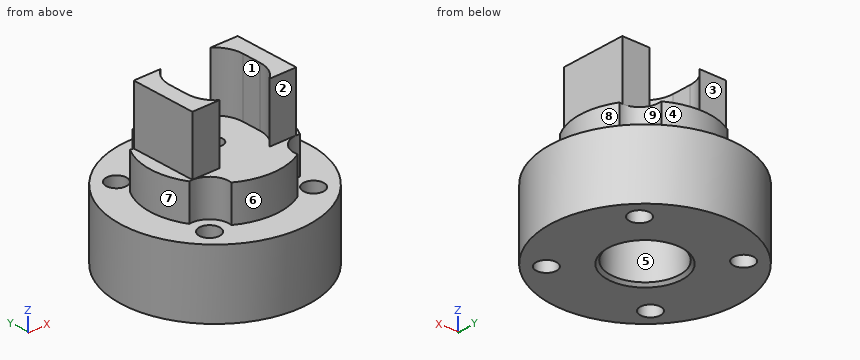
```python
from build123d import *

# Parameters (mm, degrees)
SKIZZE1_R                       = 6.7
AUFSATZ_LINEAR_AUSTRAGEN1_DEPTH = 3.75
SKIZZE1_7_R                     = 9.75
SKIZZE1_7_R_2                   = 3.55
AUFSATZ_LINEAR_AUSTRAGEN2_DEPTH = 7
SKIZZE5_R                       = 1.05
SCHNITT_LINEAR_AUSTRAGEN1_DEPTH = 11.75
SKIZZE5_3_R                     = 2
SKIZZE5_3_R_2                   = 1.05
SCHNITT_LINEAR_AUSTRAGEN2_DEPTH = 3.75
FASE1_SIZE                      = 0.3
AUFSATZ_LINEAR_AUSTRAGEN4_DEPTH = 6
M2_GEWINDEBOHRUNG1_D            = 1.6


with BuildPart() as part:
    # Skizze1 → Aufsatz-Linear austragen1 (new body)
    with BuildSketch(Plane.XY):
        Circle(SKIZZE1_R)
    extrude(amount=AUFSATZ_LINEAR_AUSTRAGEN1_DEPTH)

    # Skizze1<7> → Aufsatz-Linear austragen2 (add)
    with BuildSketch(Plane.XY):
        Circle(SKIZZE1_7_R)
        Circle(SKIZZE1_7_R_2, mode=Mode.SUBTRACT)
    extrude(amount=-AUFSATZ_LINEAR_AUSTRAGEN2_DEPTH)

    # Skizze5 → Schnitt-Linear austragen1 (cut, through all)
    with BuildSketch(Plane.XY.offset(3.75)):
        with Locations((5.409366876, 5.409366876)):
            Circle(SKIZZE5_R)
        with Locations((5.409366876, -5.409366876)):
            Circle(SKIZZE5_R)
        with Locations((-5.409366876, -5.409366876)):
            Circle(SKIZZE5_R)
        with Locations((-5.409366876, 5.409366876)):
            Circle(SKIZZE5_R)
    extrude(amount=-SCHNITT_LINEAR_AUSTRAGEN1_DEPTH, mode=Mode.SUBTRACT)

    # Skizze5<3> → Schnitt-Linear austragen2 (cut)
    with BuildSketch(Plane.XY.offset(3.75)):
        with Locations((-5.409366876, 5.409366876)):
            Circle(SKIZZE5_3_R)
        with Locations((-5.409366876, 5.409366876)):
            Circle(SKIZZE5_3_R_2, mode=Mode.SUBTRACT)
        with Locations((5.409366876, 5.409366876)):
            Circle(SKIZZE5_3_R)
        with Locations((5.409366876, 5.409366876)):
            Circle(SKIZZE5_3_R_2, mode=Mode.SUBTRACT)
        with Locations((5.409366876, -5.409366876)):
            Circle(SKIZZE5_3_R)
        with Locations((5.409366876, -5.409366876)):
            Circle(SKIZZE5_3_R_2, mode=Mode.SUBTRACT)
        with Locations((-5.409366876, -5.409366876)):
            Circle(SKIZZE5_3_R)
        with Locations((-5.409366876, -5.409366876)):
            Circle(SKIZZE5_3_R_2, mode=Mode.SUBTRACT)
    extrude(amount=-SCHNITT_LINEAR_AUSTRAGEN2_DEPTH, mode=Mode.SUBTRACT)

    # Fase1
    fase1_edges = [part.edges().sort_by_distance(p)[0] for p in [
        (-3.55, 0, -7),
    ]]
    chamfer(fase1_edges, length=FASE1_SIZE)

    # Skizze7 → Aufsatz-Linear austragen4 (add)
    with BuildSketch(Plane.XY.offset(3.75)):
        with BuildLine():
            Line((-5.4, 3.4), (-2.6, 3.4))
            ThreePointArc((-2.6, 3.4), (-3.483281573, 2.341640786), (-3.8, 1))
            Line((-3.8, 1), (-3.8, -1))
            ThreePointArc((-3.8, -1), (-3.483281573, -2.341640786), (-2.6, -3.4))
            Line((-2.6, -3.4), (-5.4, -3.4))
            Line((-5.4, -3.4), (-5.4, 3.4))
        make_face()
        with BuildLine():
            Line((5.4, -3.4), (2.6, -3.4))
            ThreePointArc((2.6, -3.4), (3.483281573, -2.341640786), (3.8, -1))
            Line((3.8, -1), (3.8, 1))
            ThreePointArc((3.8, 1), (3.483281573, 2.341640786), (2.6, 3.4))
            Line((2.6, 3.4), (5.4, 3.4))
            Line((5.4, 3.4), (5.4, -3.4))
        make_face()
    extrude(amount=AUFSATZ_LINEAR_AUSTRAGEN4_DEPTH)

    # M2 Gewindebohrung1 (through all)
    with Locations(Plane.XY.offset(3.75)):
        with Locations((0, 0)):
            Hole(M2_GEWINDEBOHRUNG1_D / 2)


solid = part.part
```
Can you work these out from the model? Positions are in its coordinate system, mm. Face numbers are marked on the shaded views. A direction names the side the tool comes from. Give positions to 0.01 mm unless a question says otherwise; leave off trailing zeros. Order: outer loops, then holes, each group sorted by start corner. A loop starts at its lowest first (then second) coordinate and runs counter-clockwise, first axis right, second up. Notation, with made-up numbers: (67.5, 0) - (87.5, 0) arc R22 cw to (87.5, 21) - close; hole circle Ø5 at (20.5, -1). An arc over 180 degrees is marked (long way). Use a Markdown table: item, result. Add a question column.
Q1. If we section it at C-C on y = 0: Write out the boundary of the cut face in (x, z).
Q2. I'm going to push flat-ended pins straight in: pin 1 (1.5 mm diameter, centred on y = -5.5, z = -2.5, fed in from +X); pin 2 (6 mm diameter, centred on x = 5, z = 3.5, fed in from +Y); pin 3 (2 mm diameter, centred on x = 4, z = 6, fed in from +Y). Where does each tip first touch, or does it pass through?
Q3. If we section it at A-A on z = 4.75: Write out the boundary of the cut face in (x, y).
Q4. If we mould it in two halves opening along X, with no side actions, what happens to the marked faces 6, 7, 8 and 9? For each: released by +X, released by -X, zero draft, split by the parting line, or undercut.
Q5. If we section it at B-B on x = 0: Write out the boundary of the cut face in (y, z), plus the area to 3 significant figures.
Q6. Please list where these lines run through material, in increasing order: line 1 along Z through (x, y) = (-2, 6.5); line 2 along Y through (x, z) = (0, -3.75); line 3 along Y through (x, z) = (5.25, 0.25).
Q7. If we section it at D-D on z = 0.75: Write out the boundary of the cut face in (x, y), plus the area to 3 significant figures.
Q8. On a 3-axis mill with a long thin cutter (end or side, diameter ignored), from which of +Z, -Z, +X, -X, +Y, -Y can I reach the whole of each face in a straight line? I mean the marked faces 1, 2, 3, 4 and 5. Say none if no direction works.
Answers follow:
| question | item | result |
|---|---|---|
| 1 | outline | (-9.75, -7) - (-3.85, -7) - (-3.55, -6.7) - (-3.55, 0) - (-0.8, 0) - (-0.8, 3.75) - (-3.8, 3.75) - (-3.8, 9.75) - (-5.4, 9.75) - (-5.4, 3.75) - (-6.7, 3.75) - (-6.7, 0) - (-9.75, 0) - close; (0.8, 0) - (3.55, 0) - (3.55, -6.7) - (3.85, -7) - (9.75, -7) - (9.75, 0) - (6.7, 0) - (6.7, 3.75) - (5.4, 3.75) - (5.4, 9.75) - (3.8, 9.75) - (3.8, 3.75) - (0.8, 3.75) - close |
| 2 | pin 1 | stops at x = 8.51 |
| 2 | pin 2 | stops at y = 6.39 |
| 2 | pin 3 | stops at y = 3.4 |
| 3 | outline | (-5.4, -3.4) - (-2.6, -3.4) arc R3 cw to (-3.8, -1) - (-3.8, 1) arc R3 cw to (-2.6, 3.4) - (-5.4, 3.4) - close; (2.6, -3.4) - (5.4, -3.4) - (5.4, 3.4) - (2.6, 3.4) arc R3 cw to (3.8, 1) - (3.8, -1) arc R3 cw to start |
| 4 | face 6 | split by the parting line |
| 4 | face 7 | released by -X |
| 4 | face 8 | released by +X |
| 4 | face 9 | undercut |
| 5 | outline | (-9.75, -7) - (-3.85, -7) - (-3.55, -6.7) - (-3.55, 0) - (-0.8, 0) - (-0.8, 3.75) - (-6.7, 3.75) - (-6.7, 0) - (-9.75, 0) - close; (0.8, 0) - (3.55, 0) - (3.55, -6.7) - (3.85, -7) - (9.75, -7) - (9.75, 0) - (6.7, 0) - (6.7, 3.75) - (0.8, 3.75) - close |
| 5 | area | 131 mm^2 |
| 6 | line 1 | z = -7 to 0 |
| 6 | line 2 | y = -9.75 to -3.55, 3.55 to 9.75 |
| 6 | line 3 | y = -3.42 to 3.42 |
| 7 | outline | (-5.75, -3.44) arc R2 cw to (-3.44, -5.75) arc R6.7 ccw to (3.44, -5.75) arc R2 cw to (5.75, -3.44) arc R6.7 ccw to (5.75, 3.44) arc R2 cw to (3.44, 5.75) arc R6.7 ccw to (-3.44, 5.75) arc R2 cw to (-5.75, 3.44) arc R6.7 ccw to start; hole circle Ø1.6 at (0, 0) |
| 7 | area | 129 mm^2 |
| 8 | face 1 | +Z |
| 8 | face 2 | +Z, +X, -X, -Y |
| 8 | face 3 | +Z, +X, -X, +Y |
| 8 | face 4 | +Z, +Y |
| 8 | face 5 | -Z |
